```python
from build123d import *

# Parameters (mm, degrees)
F0_R          = 7.5
F1_DEPTH      = 7.7
F1_DEPTH_BACK = 7.7
F2_R          = 2
F3_DEPTH      = 25
F4_R          = 7.5
F4_R_2        = 4
F5_DEPTH      = 12.2
F5_DEPTH_BACK = 12.2


with BuildPart() as f1:
    # F0 (on Front) → F1 (new body, two sides)
    with BuildSketch(Plane.XZ) as f1_sk:
        Polygon((-4, -10.5), (4, -10.5), (9, -7.5), (16, -7.5), (16, 2.5), (17, 3.5), (17, 10.5), (-17, 10.5), (-17, 3.5), (-16, 2.5), (-16, -7.5), (-9, -7.5), align=None)
        Circle(F0_R, mode=Mode.SUBTRACT)
    extrude(amount=F1_DEPTH)
    extrude(f1_sk.sketch, amount=-F1_DEPTH_BACK)

    # F2 (on face) → F3 (cut)
    with BuildSketch(Plane.XY.offset(10.5)):
        with Locations((-12, 0)):
            Circle(F2_R)
        with Locations((12, 0)):
            Circle(F2_R)
    extrude(amount=-F3_DEPTH, mode=Mode.SUBTRACT)

    # F4 (on Front) → F5 (join, two sides)
    with BuildSketch(Plane.XZ) as f5_sk:
        Circle(F4_R)
        Circle(F4_R_2, mode=Mode.SUBTRACT)
    extrude(amount=F5_DEPTH)
    extrude(f5_sk.sketch, amount=-F5_DEPTH_BACK)


solid = f1.part
```
Input: part model. Units: mm. Frame: model coordinates. A direction names the side the tool comes from. Give positions to 0.01 mm unless a question says otherwise; leave off trailing zeros. Order: outer loops, then holes, each group sorted by start corner. A loop starts at its lowest first (then second) coordinate and runs counter-clockwise, first axis right, second up. Notation, with made-up numbers: M 3,66 L 47,66 A23 cw 47,85 Z; hole C 51,66.25 d6. An arc over 180 degrees is marked long. One line per question, with ' | ' between items. Start each with the question number.
1. Access query for faces 1 (the face through (-16, 0, -2)), 2 (the face through (-4, -7.7, 7)), 3 (the face through (-7.493, 9.918, 0.33)), 4 (the face through (13, -2, -7.5)). Directions: +Z, -Z, +X, -X, +Y, -Y. A direction counts if a zero-diameter tool reaches every point of the face in a straight line with its end or side. Return the directions, or none.
2. Section query D-D (x = 0). Return the cut outline in (y, z).
3. Pull-direction query (Y, two-part tool) for faces 5 (the face through (-13.6, -1.2, 1.6)), 6 (the face through (3, 12.2, -3)), 7 (the face through (16, 0, -3)), 8 (the face through (10.4, -1.2, 1.6)); classes: released by +Y, released by -Y, zero draft, split by the parting line, or undercut.
4. Section query B-B (x = 12). Return the cut outline in (y, z), and give its area (3 significant figures).
5. Section query C-C (y = -5.25). Return the cut outline in (x, z), and give its area (3 significant figures).
6. First-contact query: pin 1 Ø2 at (y, z) = (-0.5, -0.5) entering from -X; pin 2 Ø4 at (y, z) = (8, 6) entering from -X; pin 3 Ø4 at (x, z) = (-10.5, 6) entering from +Y; pin 4 Ø5 at (x, y) = (-12, 0) entering from -Z. Flat tips, straight axial feed; report the tip coordinate or a pass-through.
7. Section query A-A (z = 0). Return the cut outline in (x, y), and give its area (3 significant figures).
8. Material intervals for probe 1 along Y at (x, z) = (-12, -0.5); probe 2 along Z at (x, y) = (0, 3.5); probe 3 along Z at (x, y) = (0, -9.5), sorted ascending. Write a range as [from, to].
Here are the results:
1) face 1: -Z, -X, +Y, -Y | face 2: -Y | face 3: +Y | face 4: -Z, +X, +Y, -Y
2) outline: M -12.2,-7.5 L -7.7,-7.5 L -7.7,-10.5 L 7.7,-10.5 L 7.7,-7.5 L 12.2,-7.5 L 12.2,-4 L -12.2,-4 Z; M -12.2,4 L 12.2,4 L 12.2,7.5 L 7.7,7.5 L 7.7,10.5 L -7.7,10.5 L -7.7,7.5 L -12.2,7.5 Z
3) face 5: undercut | face 6: released by +Y | face 7: zero draft | face 8: undercut
4) outline: M -7.7,-7.5 L -2,-7.5 L -2,10.5 L -7.7,10.5 Z; M 2,-7.5 L 7.7,-7.5 L 7.7,10.5 L 2,10.5 Z | area: 205 mm²
5) outline: M -17,3.5 L -16,2.5 L -16,-7.5 L -9,-7.5 L -4,-10.5 L 4,-10.5 L 9,-7.5 L 16,-7.5 L 16,2.5 L 17,3.5 L 17,10.5 L -17,10.5 Z; hole C 0,0 d8 | area: 580 mm²
6) pin 1: x = -16 | pin 2: x = -17 | pin 3: y = 7.7 | pin 4: z = -7.5
7) outline: M -16,-7.7 L -7.5,-7.7 L -7.5,-12.2 L -4,-12.2 L -4,12.2 L -7.5,12.2 L -7.5,7.7 L -16,7.7 Z; M 4,-12.2 L 7.5,-12.2 L 7.5,-7.7 L 16,-7.7 L 16,7.7 L 7.5,7.7 L 7.5,12.2 L 4,12.2 Z; hole C -12,0 d4; hole C 12,0 d4 | area: 407 mm²
8) probe 1: [-7.7, -2], [2, 7.7] | probe 2: [-10.5, -4], [4, 10.5] | probe 3: [-7.5, -4], [4, 7.5]
